```python
from build123d import *

# Parameters (mm, degrees)
SKETCH1_W           = 25.4
SKETCH1_H           = 21.59
SKETCH1_R           = 1.397
BOSS_EXTRUDE1_DEPTH = 2.54
SKETCH2_W           = 1.524
SKETCH2_H           = 21.59
CUT_EXTRUDE1_DEPTH  = 1.27
BOSS_EXTRUDE3_DEPTH = 1.524
SKETCH8_W           = 25.4
SKETCH8_H           = 19.05
SKETCH8_R           = 1.397
BOSS_EXTRUDE4_DEPTH = 2.54
CUT_EXTRUDE2_DEPTH  = 15.24
CUT_EXTRUDE3_DEPTH  = 15.24
BOSS_EXTRUDE5_DEPTH = 6.35
CHAMFER1_SIZE       = 5.08
FILLET1_R           = 3.048


with BuildPart() as part:
    # Sketch1 → Boss-Extrude1 (new body)
    with BuildSketch(Plane.XY):
        Rectangle(SKETCH1_W, SKETCH1_H)
        with Locations((-8.509, 5.08)):
            Circle(SKETCH1_R, mode=Mode.SUBTRACT)
        with Locations((8.509, 5.08)):
            Circle(SKETCH1_R, mode=Mode.SUBTRACT)
        with Locations((8.509, -5.08)):
            Circle(SKETCH1_R, mode=Mode.SUBTRACT)
        with Locations((-8.509, -5.08)):
            Circle(SKETCH1_R, mode=Mode.SUBTRACT)
    extrude(amount=BOSS_EXTRUDE1_DEPTH)

    # Sketch2 → Cut-Extrude1 (cut)
    with BuildSketch(Plane.XY.offset(2.54)):
        Rectangle(SKETCH2_W, SKETCH2_H)
    extrude(amount=-CUT_EXTRUDE1_DEPTH, mode=Mode.SUBTRACT)

    # Sketch7 → Boss-Extrude3 (add)
    with BuildSketch(Plane.XZ.offset(10.795)):
        Polygon((-0.762, 2.54), (-12.7, 2.54), (-12.7, 0), (12.7, 0), (12.7, 2.54), (0.762, 2.54), (0.762, 1.27), (-0.762, 1.27), align=None)
    extrude(amount=BOSS_EXTRUDE3_DEPTH)

    # Sketch8 → Boss-Extrude4 (add)
    with BuildSketch(Plane.XZ.offset(12.319)):
        with Locations((0, 3.048)):
            Rectangle(SKETCH8_W, SKETCH8_H)
        with Locations(Location((-8.89, 8.763, 0), (0, 0, 270))):
            Circle(SKETCH8_R, mode=Mode.SUBTRACT)
        with Locations(Location((8.89, 8.763, 0), (0, 0, 270))):
            Circle(SKETCH8_R, mode=Mode.SUBTRACT)
        with Locations(Location((-8.89, -2.667, 0), (0, 0, 270))):
            Circle(SKETCH8_R, mode=Mode.SUBTRACT)
        with Locations(Location((8.89, -2.667, 0), (0, 0, 270))):
            Circle(SKETCH8_R, mode=Mode.SUBTRACT)
    extrude(amount=BOSS_EXTRUDE4_DEPTH)

    # Sketch5 → Cut-Extrude2 (cut)
    with BuildSketch(Plane(origin=(0, -1.905, 0), x_dir=(-1, 0, 0), z_dir=(0, -1, 0))):
        Polygon((-4.445, -2.54), (-4.445, -5.334), (4.445, -5.334), (4.445, -2.54), (4.699, -2.54), (4.699, -5.588), (-4.699, -5.588), (-4.699, -2.54), align=None)
    extrude(amount=CUT_EXTRUDE2_DEPTH, mode=Mode.SUBTRACT)

    # Sketch9 → Cut-Extrude3 (cut)
    with BuildSketch(Plane(origin=(0, -12.319, 0), x_dir=(1, 0, 0), z_dir=(0, 1, 0))):
        Polygon((-0.762, -1.27), (0.762, -1.27), (0.762, -2.54), (4.445, -2.54), (4.445, -5.334), (-4.445, -5.334), (-4.445, -2.54), (-0.762, -2.54), align=None)
    extrude(amount=-CUT_EXTRUDE3_DEPTH, mode=Mode.SUBTRACT)

    # Sketch11 → Boss-Extrude5 (add)
    with BuildSketch(Plane(origin=(0, 1.651, 0), x_dir=(1, 0, 0), z_dir=(0, 1, 0))):
        Polygon((-4.699, -2.54), (-5.461, -2.54), (-5.461, -6.35), (5.461, -6.35), (5.461, -2.54), (4.699, -2.54), (4.699, -5.588), (-4.699, -5.588), align=None)
    extrude(amount=BOSS_EXTRUDE5_DEPTH)

    # Chamfer1
    chamfer1_edges = [part.edges().sort_by_distance(p)[0] for p in [
        (-12.7, 10.795, 1.27),
        (12.7, 10.795, 1.27),
    ]]
    chamfer(chamfer1_edges, length=CHAMFER1_SIZE)

    # Fillet1
    fillet1_edges = [part.edges().sort_by_distance(p)[0] for p in [
        (-12.7, -13.589, 12.573),
        (-12.7, -13.589, -6.477),
        (12.7, -13.589, -6.477),
        (12.7, -13.589, 12.573),
    ]]
    fillet(fillet1_edges, radius=FILLET1_R)


solid = part.part
```
Work out the finished part from the listing and answer in its coordinate system (mm). A direction names the side the tool comes from. Give positions to 0.01 mm unless a question says otherwise; leave off trailing zeros. Order: outer loops, then holes, each group sorted by start corner. A loop starts at its lowest first (then second) coordinate and runs counter-clockwise, first axis right, second up.
1. The mould has two halves that part along Z. Classify faces 4 (the cylindrical face through (-11.83, -13.61, 11.66)), 5 (the cylindrical face through (-9.62, 4.23, 1.25)), 6 (the flat face through (-0.762, -2, 2)): released by +Z, released by -Z, zero draft, split by the parting line, or undercut.
Result sheet:
face 4: released by +Z
face 5: zero draft
face 6: undercut
2. For faces 1 (the flat face through (0, 1.651, 6)), 2 (the flat face through (0, -14, 5.588)), 3 (the flat face through (0, -1, 0)), determine the directions among +Z, -Z, +X, -X, +Y, -Y from which every point of the face is accessible in a straight line to the end or side of a thin tool.
Result sheet:
face 1: +Z, +X, -X
face 2: +Y, -Y
face 3: -Z, +X, -X, +Y
3. Straight lines are drawn through the part: L1, parallel to X at y = 6, z = 4; L2, parallel to X at y = -5.5, z = 1; L3, parallel to Y at x = 11.25, z = -1.75. For each, find the intervals that lie inside material, in ascending order.
Result sheet:
L1: x = -5.46 to -4.7, 4.7 to 5.46
L2: x = -12.7 to -9.84, -7.18 to 7.18, 9.84 to 12.7
L3: y = -14.86 to -12.32
4. Section A-A, the plane y = 5.08 is taken. Determine the outline of the cut face in (x, z), and give its area (3 significant figures).
Result sheet:
outline: (-12.7, 0) - (-9.91, 0) - (-9.91, 2.54) - (-12.7, 2.54) - close; (-7.11, 0) - (7.11, 0) - (7.11, 2.54) - (5.46, 2.54) - (5.46, 6.35) - (-5.46, 6.35) - (-5.46, 2.54) - (-7.11, 2.54) - close; (9.91, 0) - (12.7, 0) - (12.7, 2.54) - (9.91, 2.54) - close; hole (-4.7, 2.54) - (-0.76, 2.54) - (-0.76, 1.27) - (0.76, 1.27) - (0.76, 2.54) - (4.7, 2.54) - (4.7, 5.59) - (-4.7, 5.59) - close
area: 61.4 mm2
5. Section B-B, the plane z = 0.75 is taken. Determine the outline of the cut face in (x, y) (3 decimals), and give its area (3 significant figures).
Result sheet:
outline: (-12.7, -14.859) - (12.7, -14.859) - (12.7, 5.715) - (7.62, 10.795) - (-7.62, 10.795) - (-12.7, 5.715) - close; hole circle Ø2.794 at (-8.509, -5.08); hole circle Ø2.794 at (-8.509, 5.08); hole circle Ø2.794 at (8.509, -5.08); hole circle Ø2.794 at (8.509, 5.08)
area: 601 mm2
6. Section C-C, the plane y = -5.08 is taken. Determine the outline of the cut face in (x, z), and give its area (3 significant figures).
Result sheet:
outline: (-12.7, 0) - (-9.91, 0) - (-9.91, 2.54) - (-12.7, 2.54) - close; (-7.11, 0) - (7.11, 0) - (7.11, 2.54) - (0.76, 2.54) - (0.76, 1.27) - (-0.76, 1.27) - (-0.76, 2.54) - (-7.11, 2.54) - close; (9.91, 0) - (12.7, 0) - (12.7, 2.54) - (9.91, 2.54) - close
area: 48.4 mm2
7. Section D-D, the plane x = -8.89 is taken. Determine the outline of the cut face in (y, z) (3 decimals).
Result sheet:
outline: (-14.859, -6.477) - (-12.319, -6.477) - (-12.319, -4.064) - (-14.859, -4.064) - close; (-14.859, -1.27) - (-12.319, -1.27) - (-12.319, 0) - (-6.424, 0) - (-6.424, 2.54) - (-12.319, 2.54) - (-12.319, 7.366) - (-14.859, 7.366) - close; (-14.859, 10.16) - (-12.319, 10.16) - (-12.319, 12.573) - (-14.859, 12.573) - close; (-3.736, 0) - (3.736, 0) - (3.736, 2.54) - (-3.736, 2.54) - close; (6.424, 0) - (9.525, 0) - (9.525, 2.54) - (6.424, 2.54) - close
8. Each of these flat-tipped pins is pushed along its axis until it touches: P1, Ø1, axis at x = -1.5, y = -11, coming from the -Z side; P2, Ø5, axis at x = 9.5, y = -10, coming from the +Z side; P3, Ø1.5, axis at x = 4.5, y = 6, coming from the +Z side; P4, Ø1.5, axis at y = 6, z = 4, coming from the +X side. Where does it stop, or does it pass through?
Result sheet:
P1: stops at z = 0
P2: stops at z = 12.57
P3: stops at z = 6.35
P4: stops at x = 5.46
